Verification items for the finished model (mm, model axes). A direction names the side the tool comes from. Coordinates: 2 decimals unless noted, no trailing zeros. Write each loop counter-clockwise with the first axis right and the second up, starting at its lowest first coordinate (ties: lowest second). Pieces come first, ordered by that corner, then holes. Notation, with made-up numbers: (77.25, -4) -> (127.25, -4) arc R22 ccw to (127.25, 8) -> close; hole circle Ø9 at (26.5, -9.5). An arc over 180 degrees is marked (long way). Answer in a Markdown table with one row per item.
```python
from build123d import *

# Parameters (mm, degrees)
BOSS_EXTRU_1_DEPTH = 10.3
D_GAGEMENT_M41_D   = 4.5


with BuildPart() as part:
    # Esquisse1 → Boss.-Extru.1 (new body)
    with BuildSketch(Plane.XY):
        Polygon((0, 0), (0, 2), (2, 2), (-1, 5), (-5, 5), (-8, 2), (-6, 2), (-6, 0), align=None)
    extrude(amount=BOSS_EXTRU_1_DEPTH)

    # Dégagement M41 (through all)
    with Locations(Plane(origin=(0, 5, 0), x_dir=(1, 0, 0), z_dir=(0, 1, 0))):
        with Locations((-3, -5.15)):
            Hole(D_GAGEMENT_M41_D / 2)


solid = part.part
```
1. Release check for a two-part mould opening along X. For faces 1 (the face through (-2.71, 2.46, 2.92)), 2 (the face through (-3, 5, 2)), 3 (the face through (1, 3, 5)), 4 (the face through (-6, 1, 5)) record: released by +X, released by -X, zero draft, split by the parting line, or undercut.
Findings below:
| item | result |
|---|---|
| face 1 | undercut |
| face 2 | zero draft |
| face 3 | released by +X |
| face 4 | released by -X |
2. Sectioned sample at B-B, the plane y = 2.35. Record the cut outline in (x, z), and give its area (3 significant figures).
Findings below:
| item | result |
|---|---|
| outline | (-7.65, 0) -> (1.65, 0) -> (1.65, 10.3) -> (-7.65, 10.3) -> close; hole circle Ø4.5 at (-3, 5.15) |
| area | 79.9 mm² |
3. Sectioned sample at A-A, the plane x = -3. Record the cut outline in (y, z), and give its area (3 significant figures).
Findings below:
| item | result |
|---|---|
| outline | (0, 0) -> (5, 0) -> (5, 2.9) -> (0, 2.9) -> close; (0, 7.4) -> (5, 7.4) -> (5, 10.3) -> (0, 10.3) -> close |
| area | 29.0 mm² |
4. Material ranges on probe 1 along Z at (x, y) = (-3, 1.3); probe 2 along Z at (x, y) = (-5, 4.2); probe 3 along X at (y, z) = (0.45, 4.75), recorded low to high. Write a range as from..to.
Findings below:
| item | result |
|---|---|
| probe 1 | z = 0..2.9, 7.4..10.3 |
| probe 2 | z = 0..4.12, 6.18..10.3 |
| probe 3 | x = -6..-5.21, -0.79..0 |
5. Access from +Z, -Z, +X, -X, +Y, -Y to the whole of each face (thin tool, end or side, straight path). Record for faces 5 (the face through (0, 1, 5)), 6 (the face through (-6, 4, 5)), 7 (the face through (-7, 2, 5)).
Findings below:
| item | result |
|---|---|
| face 5 | +Z, -Z, +X, -Y |
| face 6 | +Z, -Z, -X, +Y |
| face 7 | +Z, -Z, -X, -Y |
6. Sectioned sample at C-C, the plane z = 8. Record the cut outline in (x, y).
Findings below:
| item | result |
|---|---|
| outline | (-8, 2) -> (-6, 2) -> (-6, 0) -> (0, 0) -> (0, 2) -> (2, 2) -> (-1, 5) -> (-5, 5) -> close |
7. Go/stop test with flat-tipped pins: pin 1 (1.5 mm diameter, centred on y = 4, z = 7, fed in from -X); pin 2 (2 mm diameter, centred on x = -6.5, z = 5.5, fed in from -Y); pin 3 (1 mm diameter, centred on y = 3, z = 2.5, fed in from +X); pin 4 (1.6 mm diameter, centred on x = 1, z = 5.5, fed in from -Y). Record where each tip stops, or that it passes through.
Findings below:
| item | result |
|---|---|
| pin 1 | stops at x = -6.75 |
| pin 2 | stops at y = 0 |
| pin 3 | stops at x = 1.5 |
| pin 4 | stops at y = 2 |
8. Sectioned sample at D-D, the plane z = 3.5. Record the cut outline in (x, y), and give its area (3 significant figures).
Findings below:
| item | result |
|---|---|
| outline | (-8, 2) -> (-6, 2) -> (-6, 0) -> (-4.53, 0) -> (-4.53, 5) -> (-5, 5) -> close; (-1.47, 0) -> (0, 0) -> (0, 2) -> (2, 2) -> (-1, 5) -> (-1.47, 5) -> close |
| area | 17.7 mm² |
